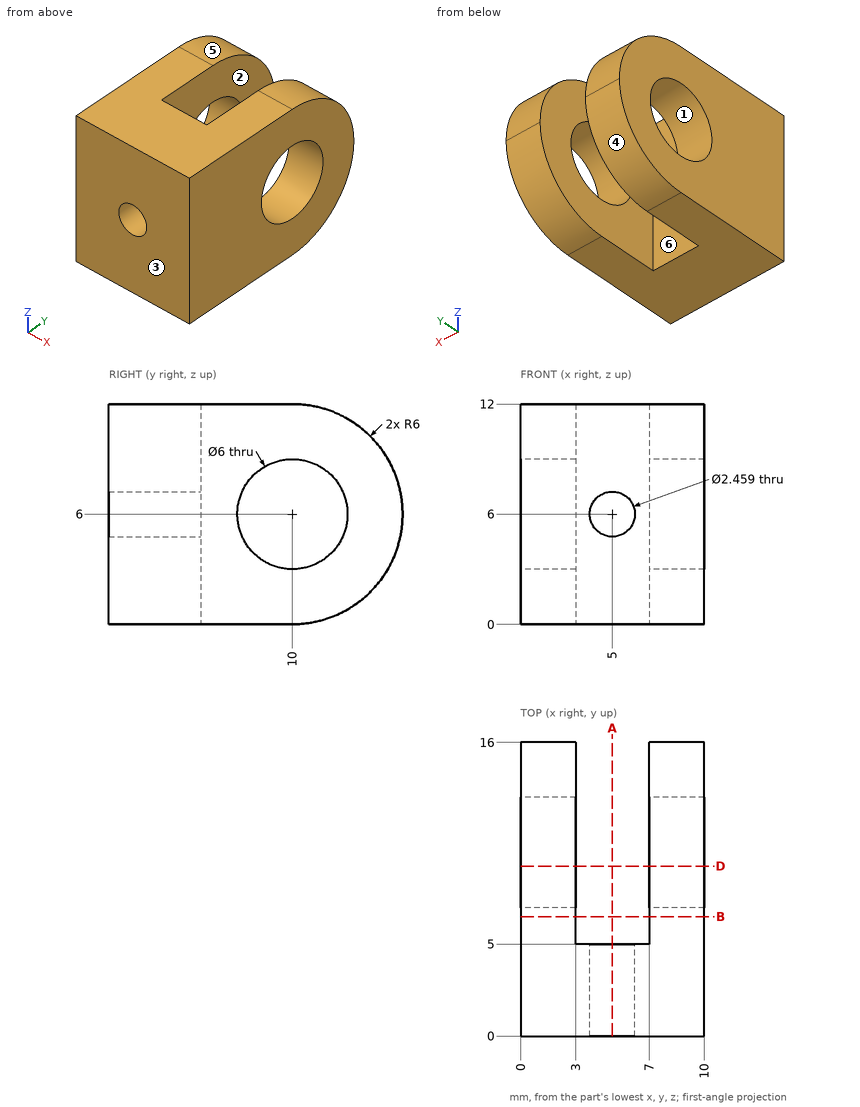
The figure shows three views and two pictorial views of one solid part (mm, origin at its lowest corner). Answer the questions. A direction names the side the tool comes from. Round coordinates to 2 decimals unless told otherwise and drop trailing zeros. Loops run counter-clockwise (first coordinate to the right, second up) from the corner with the lowest first, then second, coordinate; pieces in that order, holes last. Notation, with made-up numbers: (-27, -6) - (21, -6) arc R20 ccw to (21, 27) - close; hole circle Ø4 at (-12, -24). An arc over 180 degrees is marked (long way). Use one line per item in the form item = value. Start each with the question number.
(1) Find section B-B on y = 6.5. Determine the outline of the cut face in (x, z).
(2) Flat-ended cylindrical pins translate along their axes: P1, Ø1.5, axis at x = 5, y = 13, coming from the +Z side; P2, Ø2, axis at x = 3, z = 4.5, coming from the +Y side; P3, Ø2, axis at x = 5, z = 3.5, coming from the +Y side. Find the tip coordinate at first contact, or state that the pin passes through.
(3) Determine the mould class of the marked faces 1, 2, 3 and 4 for opening direction Y: +Y half, -Y half, draft (parallel to the pull), parting line (faces both ways), or undercut.
(4) Find section D-D on y = 9.25. Determine the outline of the cut face in (x, z) (1 decimal).
(5) Find section A-A on x = 5. Determine the outline of the cut face in (y, z).
(6) Consider line 1 (Y direction, x = 1.85, z = 6); line 2 (X direction, y = 7, z = 9); line 3 (X direction, y = 3.9, z = 6). Determine where each line is inside the solid, lowest interval first.
(7) Which of the six approach directions +Z, -Z, +X, -X, +Y, -Y give full straight-line access (tool end or side, diameter ignored) to the marked faces 5 and 6?
Answer list:
q1.outline = (0, 0) - (3, 0) - (3, 12) - (0, 12) - close; (7, 0) - (10, 0) - (10, 12) - (7, 12) - close
q2.P1 = through
q2.P2 = 15.98
q2.P3 = 5
q3.face_1 = undercut
q3.face_2 = draft
q3.face_3 = -Y half
q3.face_4 = +Y half
q4.outline = (0, 0) - (3, 0) - (3, 3.1) - (0, 3.1) - close; (0, 8.9) - (3, 8.9) - (3, 12) - (0, 12) - close; (7, 0) - (10, 0) - (10, 3.1) - (7, 3.1) - close; (7, 8.9) - (10, 8.9) - (10, 12) - (7, 12) - close
q5.outline = (0, 0) - (5, 0) - (5, 4.77) - (0, 4.77) - close; (0, 7.23) - (5, 7.23) - (5, 12) - (0, 12) - close
q6.line_1 = 0 to 7, 13 to 16
q6.line_2 = 0 to 3, 7 to 10
q6.line_3 = 0 to 3.77, 6.23 to 10
q7.face_5 = +Z, +X, -X, +Y
q7.face_6 = +Z, -Z, +Y
